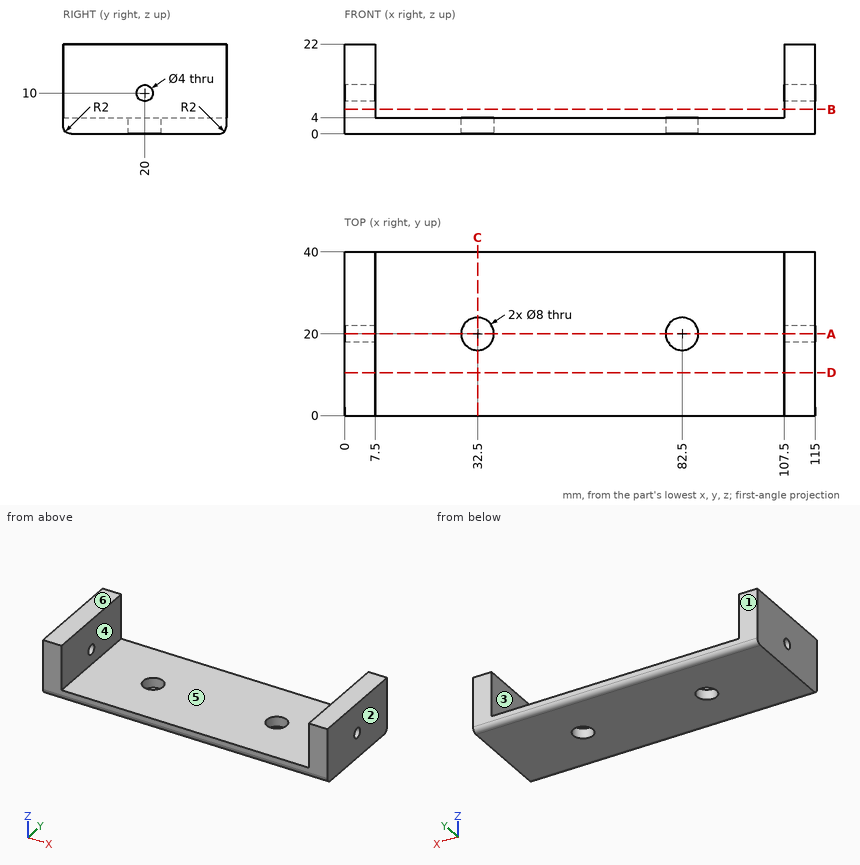
For this review, use the dimensioned drawing (mm, ordinates from the lowest corner) and the shaded views. A direction names the side the tool comes from. Coordinates: 2 decimals unless noted, no trailing zeros. Loops run counter-clockwise (first coordinate to the right, second up) from the corner with the lowest first, then second, coordinate; pieces in that order, holes last. Notation, with made-up numbers: (52, 28) - (60, 28) arc R33 cw to (60, 67) - close; hole circle Ø3 at (35, 53). An arc over 180 degrees is marked (long way). Use one line per item in the form item = value. Start each with the question number.
1) Draft analysis for pull direction X (two halves, no side actions). For the marked faces 1, 2, 3 and 4, state which applies: released by +X, released by -X, zero draft, split by the parting line, or undercut.
2) Take a section at A-A (y = 20). State the section outline as (x, z) points, plus the area to 3 significant figures.
3) For pin 1 (9 mm diameter, centred on x = 32.5, y = 20, fed in from +Z); pin 2 (3.5 mm diameter, centred on y = 20, z = 10, fed in from +X), all flat-tipped, find the tip position at first contact; note any pin that passes through.
4) Take a section at C-C (x = 32.5). State the section outline as (y, z) points.
5) To check wall thickness, follow probe 1 along X at (y, z) = (10.5, 7); probe 2 along Y at (x, z) = (82.5, 2.95); probe 3 along Z at (x, y) = (5.75, 20). State the ranges of each line that lie inside material, in increasing order. Write a range as from..to.
6) Take a section at B-B (z = 6). State the section outline as (x, y) points, plus the area to 3 significant figures.
7) Take a section at D-D (y = 10.5). State the section outline as (x, z) points, plus the area to 3 significant figures.
8) For the marked faces 5 and 6, list the 3-axis set-ups (+Z, -Z, +X, -X, +Y, -Y) from which the entire face can be reached by the end or side of a thin tool; tool diameter is ignored.
From the geometry:
q1.face_1 = zero draft
q1.face_2 = released by +X
q1.face_3 = undercut
q1.face_4 = undercut
q2.outline = (0, 0) - (28.5, 0) - (28.5, 4) - (7.5, 4) - (7.5, 8) - (0, 8) - close; (0, 12) - (7.5, 12) - (7.5, 22) - (0, 22) - close; (36.5, 0) - (78.5, 0) - (78.5, 4) - (36.5, 4) - close; (86.5, 0) - (115, 0) - (115, 8) - (107.5, 8) - (107.5, 4) - (86.5, 4) - close; (107.5, 12) - (115, 12) - (115, 22) - (107.5, 22) - close
q2.area = 606 mm2
q3.pin_1 = 4
q3.pin_2 = through
q4.outline = (0, 2) arc R2 ccw to (2, 0) - (16, 0) - (16, 4) - (0, 4) - close; (24, 0) - (38, 0) arc R2 ccw to (40, 2) - (40, 4) - (24, 4) - close
q5.probe_1 = 0..7.5, 107.5..115
q5.probe_2 = 0..16, 24..40
q5.probe_3 = 0..8, 12..22
q6.outline = (0, 0) - (7.5, 0) - (7.5, 40) - (0, 40) - close; (107.5, 0) - (115, 0) - (115, 40) - (107.5, 40) - close
q6.area = 600 mm2
q7.outline = (0, 0) - (115, 0) - (115, 22) - (107.5, 22) - (107.5, 4) - (7.5, 4) - (7.5, 22) - (0, 22) - close
q7.area = 730 mm2
q8.face_5 = +Z, +Y, -Y
q8.face_6 = +Z, +X, -X, +Y, -Y
